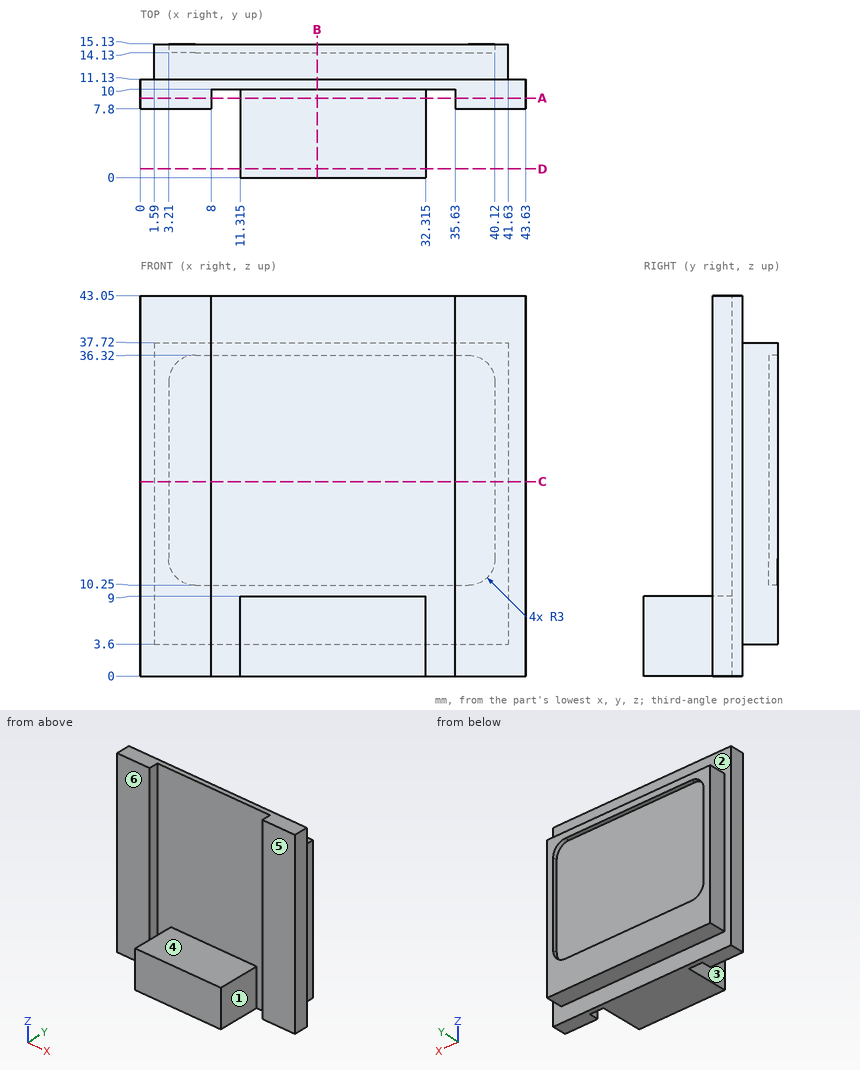
Print and shaded views of the part. All mm, measured from the part's lowest x, y and z. A direction names the side the tool comes from. Give positions to 0.01 mm unless a question says otherwise; leave off trailing zeros. Write each loop counter-clockwise with the first axis right and the second up, starting at its lowest first coordinate (ties: lowest second). Pieces come first, ordered by that corner, then holes. Notation, with made-up numbers: (-16, 5.25) -> (26, 5.25) arc R27 cw to (26, 34.25) -> close; hole circle Ø7 at (56, -3.75). An arc over 180 degrees is marked (long way). Write item = value, one per line.
(1) Probe line 1 along X through (y, z) = (9.25, 7.5) (3 decimals); line 2 along Y through (x, z) = (35, 29.5); line 3 along Z through (x, y) = (9, 11.75). List the from-to ranges inside material, lowest first.
Determined:
line_1 = 0 to 8, 11.315 to 32.315, 35.63 to 43.63
line_2 = 10 to 14.13
line_3 = 3.6 to 37.72
(2) Slice it at C-C, the plane z = 22. Give the cut face in (x, y), then the cut area to 3 significant figures.
Determined:
outline = (0, 7.8) -> (8, 7.8) -> (8, 10) -> (35.63, 10) -> (35.63, 7.8) -> (43.63, 7.8) -> (43.63, 11.13) -> (41.63, 11.13) -> (41.63, 15.13) -> (40.12, 15.13) -> (40.12, 14.13) -> (3.21, 14.13) -> (3.21, 15.13) -> (1.59, 15.13) -> (1.59, 11.13) -> (0, 11.13) -> close
area = 208 mm2
(3) Slice it at A-A, the plane y = 9. Give the cut face in (x, z) (3 decimals).
Determined:
outline = (0, 0) -> (8, 0) -> (8, 43.05) -> (0, 43.05) -> close; (11.315, 0) -> (32.315, 0) -> (32.315, 9) -> (11.315, 9) -> close; (35.63, 0) -> (43.63, 0) -> (43.63, 43.05) -> (35.63, 43.05) -> close
(4) Tool access for the marked faces 3, 4, 5 and 6: list every direction of +Z, -Z, +X, -X, +Y, -Y with a clear straight run to the whole face (end or side of a thin tool).
Determined:
face_3 = +Z, -Z, -Y
face_4 = +Z, -Y
face_5 = +Z, -Z, +X, -Y
face_6 = +Z, -Z, -X, -Y
(5) Slice it at B-B, the plane x = 20. Give the cut face in (y, z).
Determined:
outline = (0, 0) -> (11.13, 0) -> (11.13, 3.6) -> (15.13, 3.6) -> (15.13, 10.25) -> (14.13, 10.25) -> (14.13, 36.32) -> (15.13, 36.32) -> (15.13, 37.72) -> (11.13, 37.72) -> (11.13, 43.05) -> (10, 43.05) -> (10, 9) -> (0, 9) -> close
(6) Slice it at D-D, the plane y = 1. Give the cut face in (x, z) (3 decimals).
Determined:
outline = (11.315, 0) -> (32.315, 0) -> (32.315, 9) -> (11.315, 9) -> close
(7) Mould opens along X. For the marked faces 1 and 2 say: released by +X, released by -X, zero draft, split by the parting line, or undercut.
Determined:
face_1 = undercut
face_2 = zero draft
(8) Flat gauge pins, fed straight in: P1, Ø5, axis at y = 6, z = 24.5, coming from the -X side; P2, Ø5, axis at x = 15.5, z = 30.5, coming from the +Y side; P3, Ø1.2, axis at y = 14, z = 17, coming from the -X side; P4, Ø1.1, axis at x = 18.5, y = 14.5, coming from the -Z side. Where does each tip first touch, or does it go through?
Determined:
P1 = 0
P2 = 14.13
P3 = 1.59
P4 = 3.6
